```python
from build123d import *

# Parameters (mm, degrees)
BOSS_EXTRUDE4_DEPTH = 56
BOSS_EXTRUDE5_DEPTH = 24
SKETCH7_R           = 16
CUT_EXTRUDE1_DEPTH  = 40


with BuildPart() as part:
    # Sketch5 → Boss-Extrude4 (new body)
    with BuildSketch(Plane(origin=(0, 0, 0), x_dir=(1, 0, 0), z_dir=(0, 1, 0))):
        with BuildLine():
            Line((27.838821814, -3), (15.716233646, -3))
            ThreePointArc((15.716233646, -3), (-16, 0), (15.716233646, 3))
            Line((15.716233646, 3), (27.838821814, 3))
            ThreePointArc((27.838821814, 3), (-28, 0), (27.838821814, -3))
        make_face()
    extrude(amount=BOSS_EXTRUDE4_DEPTH)

    # Sketch6 → Boss-Extrude5 (add)
    with BuildSketch(Plane(origin=(0, 0, 0), x_dir=(1, 0, 0), z_dir=(0, 1, 0))):
        with BuildLine():
            Line((-90, 24), (-90, -24))
            Line((-90, -24), (-14.422205102, -24))
            ThreePointArc((-14.422205102, -24), (-28, 0), (-14.422205102, 24))
            Line((-14.422205102, 24), (-90, 24))
        make_face()
    extrude(amount=BOSS_EXTRUDE5_DEPTH)

    # Sketch7 → Cut-Extrude1 (cut)
    with BuildSketch(Plane.ZY.offset(90)):
        with Locations((0, 24)):
            Circle(SKETCH7_R)
    extrude(amount=-CUT_EXTRUDE1_DEPTH, mode=Mode.SUBTRACT)


solid = part.part
```
Check sheet for the modelled part. Datum: model origin and axes. Units: mm. A direction names the side the tool comes from. Coordinates: 2 decimals unless noted, no trailing zeros. Loops run counter-clockwise (first coordinate to the right, second up) from the corner with the lowest first, then second, coordinate; pieces in that order, holes last. Notation, with made-up numbers: M 0.5,-28 L 47.5,-28 A26 cw 47.5,7 Z; hole C 78.5,-18 d1. An arc over 180 degrees is marked long. Answer as a JSON object with one key per item and string values.
1. Scan lines: L1, parallel to Z at x = 0, y = 31; L2, parallel to Y at x = -44, z = 18.5; L3, parallel to X at y = 14, z = 0. Record each from-to range of solid material in increasing order. Write a range as from..to.
Outcome:
{"L1": "-28..-16, 16..28", "L2": "0..24", "L3": "-50..-16"}
2. Access from +Z, -Z, +X, -X, +Y, -Y to the whole of each face (thin tool, end or side, straight path). Record for faces 4 (the flat face through (22, 28, -3)), 5 (the flat face through (-90, 6, 0)), 6 (the flat face through (-50, 18, 0)), 7 (the flat face through (-52, 12, -24)), 8 (the flat face through (-53, 12, 24)).
Outcome:
{"face 4": "+X, +Y, -Y", "face 5": "+Z, -Z, -X, +Y, -Y", "face 6": "-X, +Y", "face 7": "-Z, -X, +Y, -Y", "face 8": "+Z, -X, +Y, -Y"}
3. Sectioned sample at A-A on x = 0. Record the cut outline in (y, z), and give its area (3 significant figures).
Outcome:
{"outline": "M 0,-28 L 56,-28 L 56,-16 L 0,-16 Z; M 0,16 L 56,16 L 56,28 L 0,28 Z", "area": "1,340 mm²"}
4. Depth check by flat-ended pin: P1, Ø10, axis at y = 30.5, z = 9, coming from the +X side; P2, Ø24, axis at x = -40.5, z = 1.5, coming from the +Y side; P3, Ø3, axis at y = 13, z = 8.5, coming from the -X side. Enter the tip coordinate at first touch or a pass-through.
Outcome:
{"P1": "x = 27.71", "P2": "y = 24", "P3": "x = -50"}
5. Sectioned sample at D-D on x = -54.5. Record the cut outline in (y, z), and give its area (3 significant figures).
Outcome:
{"outline": "M 0,-24 L 24,-24 L 24,-16 A16 cw 24,16 L 24,24 L 0,24 Z", "area": "750 mm²"}
6. Release check for a two-part mould opening along Z. For faces 1 (the cylindrical face through (25.768, 27.608, -10.955)), 2 (the flat face through (22, 28, 3)), 3 (the flat face through (-32, 0, 0)) record: pulls with the +Z half, pulls with the -Z half, needs draft (parallel to the pull), parting line crosses it, or undercut.
Outcome:
{"face 1": "parting line crosses it", "face 2": "undercut", "face 3": "needs draft"}
7. Sectioned sample at C-C on y = 12. Record the cut outline in (x, z), and give its area (3 significant figures).
Outcome:
{"outline": "M -90,-24 L -14.42,-24 A28 ccw 27.84,-3 L 15.72,-3 A16 cw long 15.72,3 L 27.84,3 A28 ccw -14.42,24 L -90,24 L -90,10.58 L -50,10.58 L -50,-10.58 L -90,-10.58 Z", "area": "3,910 mm²"}
8. Sectioned sample at B-B on z = 0. Record the cut outline in (x, y), and give its area (3 significant figures).
Outcome:
{"outline": "M -90,0 L -16,0 L -16,56 L -28,56 L -28,24 L -50,24 L -50,8 L -90,8 Z", "area": "1,520 mm²"}
